Here's the drawing with two shaded views (mm, measured from the low corner). I have some questions. A direction names the side the tool comes from. Coordinates: 2 decimals unless noted, no trailing zeros. Write each loop counter-clockwise with the first axis right and the second up, starting at its lowest first coordinate (ties: lowest second). Pieces come first, ordered by that corner, then holes. Notation, with made-up numbers: (35, 32) -> (62, 32) arc R22 cw to (62, 65) -> close; hole circle Ø3 at (78, 73). An arc over 180 degrees is marked (long way). Use a Markdown table: item, result. Add a question column.
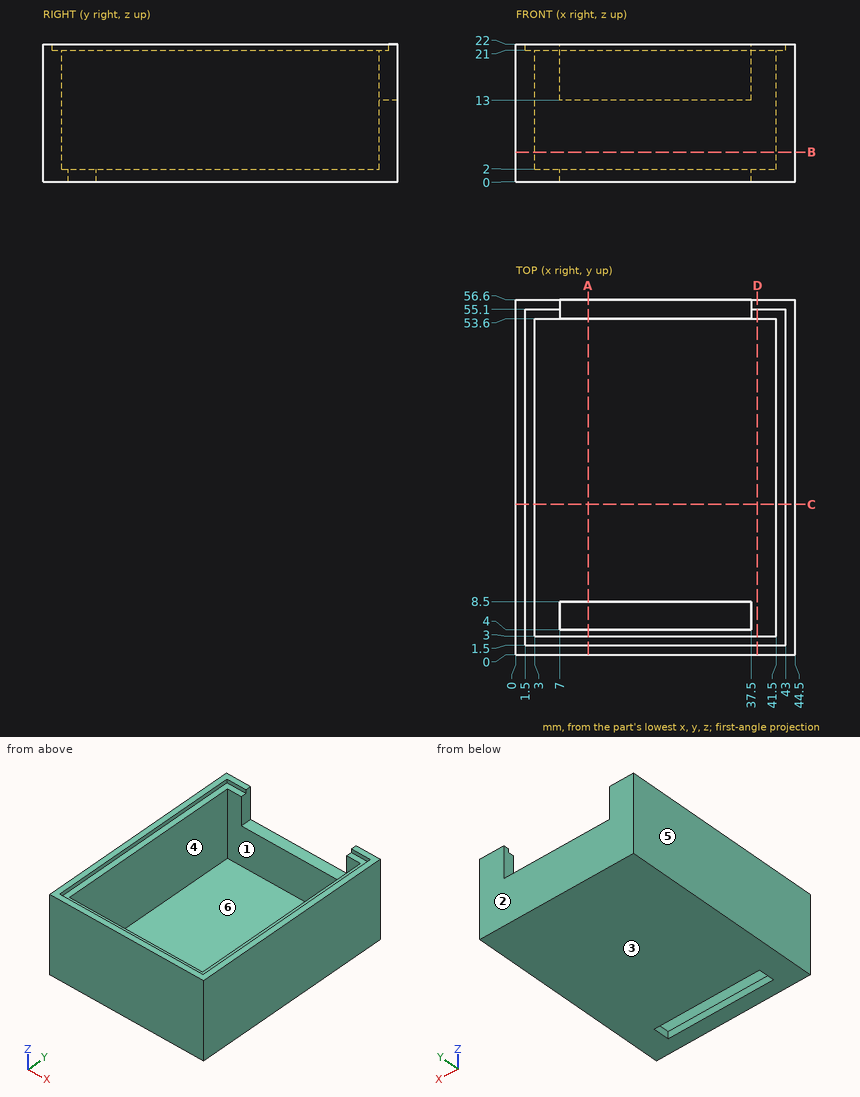
Q1. Which directions (+Z, -Z, +X, -X, +Y, -Y) give clear straight access to the entire face, cutting with the end or side of a thin tool? Please do the marked faces 5 and 6.
Q2. Suppose I cut it at D-D, the plane x = 38.5. Write out the boundary of the cut face in (y, z), and give its area (3 significant figures).
Q3. Thinking about a two-plate mould opening in Y: for the marked faces 1, 2, 3 and 4, which applies, released by +Y, released by -Y, zero draft, split by the parting line, or undercut?
Q4. Will these pins go through, and if not, where does the flat tip stop? pin 1 (2.5 mm diameter, centred on x = 16.5, y = 55.5, fed in from +Z); pin 2 (12.5 mm diameter, centred on x = 19, y = 16.5, fed in from +Z).
Q5. Suppose I cut it at C-C, the plane y = 24. Write out the boundary of the cut face in (x, z).
Q6. Suppose I cut it at B-B, the plane z = 4.75. Write out the boundary of the cut face in (x, y), and give its area (3 significant figures).
Q7. Suppose I cut it at A-A, the plane x = 11.5. Write out the boundary of the cut face in (y, z), and give its area (3 significant figures).
Q8. Please list where these lines run through material, in increasing order: line 1 (X direction, y = 40, z = 15.25); line 2 (Y direction, x = 8.5, z = 9.5); line 3 (Y direction, x = 29.5, z = 19).
Answer key:
| question | item | result |
|---|---|---|
| 1 | face 5 | +Z, -Z, -X, +Y, -Y |
| 1 | face 6 | +Z |
| 2 | outline | (0, 0) -> (56.6, 0) -> (56.6, 22) -> (55.1, 22) -> (55.1, 21) -> (53.6, 21) -> (53.6, 2) -> (3, 2) -> (3, 21) -> (1.5, 21) -> (1.5, 22) -> (0, 22) -> close |
| 2 | area | 230 mm^2 |
| 3 | face 1 | undercut |
| 3 | face 2 | released by +Y |
| 3 | face 3 | zero draft |
| 3 | face 4 | undercut |
| 4 | pin 1 | stops at z = 13 |
| 4 | pin 2 | stops at z = 2 |
| 5 | outline | (0, 0) -> (44.5, 0) -> (44.5, 22) -> (43, 22) -> (43, 21) -> (41.5, 21) -> (41.5, 2) -> (3, 2) -> (3, 21) -> (1.5, 21) -> (1.5, 22) -> (0, 22) -> close |
| 6 | outline | (0, 0) -> (44.5, 0) -> (44.5, 56.6) -> (0, 56.6) -> close; hole (3, 3) -> (41.5, 3) -> (41.5, 53.6) -> (3, 53.6) -> close |
| 6 | area | 571 mm^2 |
| 7 | outline | (0, 0) -> (4, 0) -> (4, 2) -> (3, 2) -> (3, 21) -> (1.5, 21) -> (1.5, 22) -> (0, 22) -> close; (8.5, 0) -> (56.6, 0) -> (56.6, 13) -> (53.6, 13) -> (53.6, 2) -> (8.5, 2) -> close |
| 7 | area | 196 mm^2 |
| 8 | line 1 | x = 0 to 3, 41.5 to 44.5 |
| 8 | line 2 | y = 0 to 3, 53.6 to 56.6 |
| 8 | line 3 | y = 0 to 3 |
